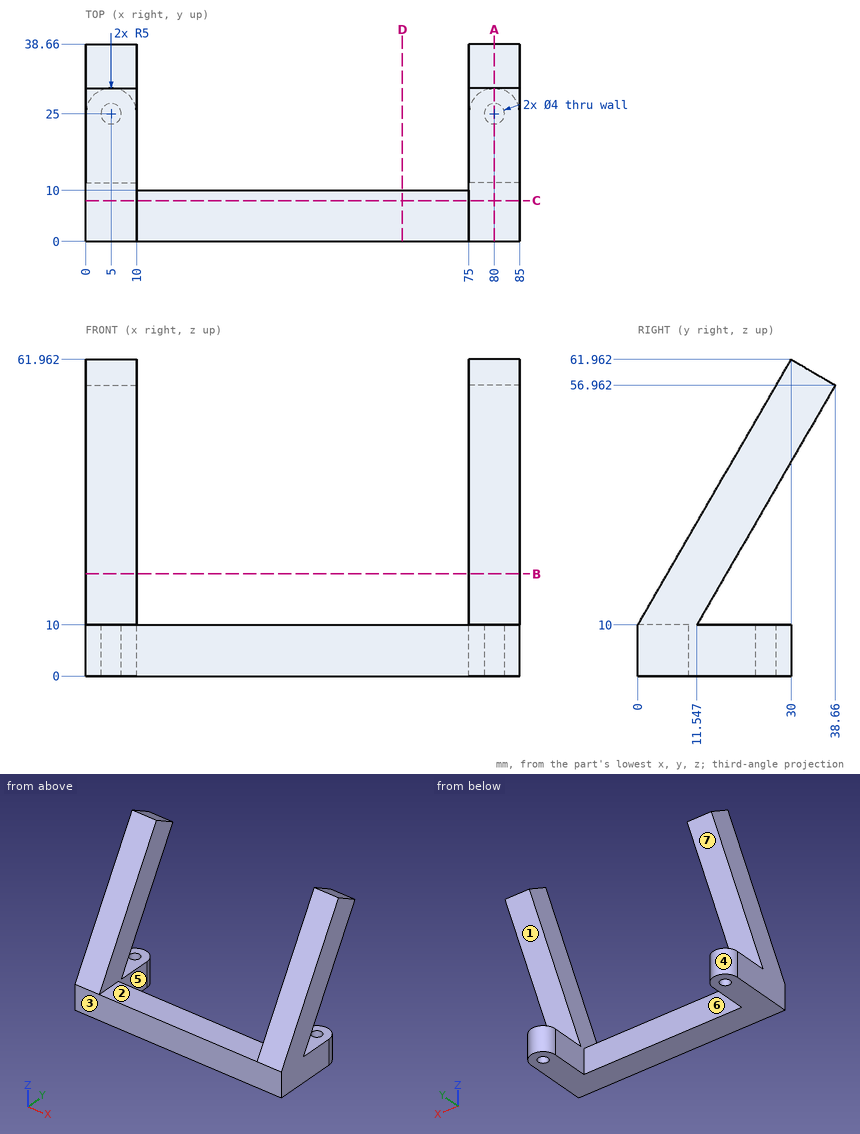
Study the drawing (mm; zero at the part's minimum x, y, z) and answer. A direction names the side the tool comes from. Coordinates: 2 decimals unless noted, no trailing zeros. Loops run counter-clockwise (first coordinate to the right, second up) from the corner with the lowest first, then second, coordinate; pieces in that order, holes last. Notation, with made-up numbers: (37.5, 35) -> (67.5, 35) arc R24 ccw to (67.5, 45) -> close; hole circle Ø8 at (66.5, 0.25). An arc over 180 degrees is marked (long way). Answer as CSV lines item,"result".
1) Flat-ended cylindrical pins translate along their axes: pin 1 (4.5 mm diameter, centred on x = 80, y = 25, fed in from +Z); pin 2 (11 mm diameter, centred on x = 43, z = 6.5, fed in from +Y); pin 3 (11 mm diameter, centred on x = 42.5, y = 3.5, fed in from +Z); pin 4 (8 mm diameter, centred on x = 38.5, z = 17.5, fed in from -Y). Find the tip coordinate at first contact, or state that the pin passes through.
A:
pin 1,"stops at z = 57.2"
pin 2,"stops at y = 10"
pin 3,"stops at z = 10"
pin 4,"passes through"
2) The part is cut by section C-C (y = 8). Give the vertices of the cut face in (x, z).
A:
outline,"(0, 0) -> (85, 0) -> (85, 23.86) -> (75, 23.86) -> (75, 10) -> (10, 10) -> (10, 23.86) -> (0, 23.86) -> close"
3) The part is cut by section D-D (x = 62). Give the vertices of the cut face in (y, z).
A:
outline,"(0, 0) -> (10, 0) -> (10, 10) -> (0, 10) -> close"
4) For a pull along Z with two mould halves and no side action, classify the marked faces 1, 2 and 3 as released by +Z, released by -Z, zero draft, split by the parting line, or undercut.
A:
face 1,"undercut"
face 2,"released by +Z"
face 3,"zero draft"
5) The part is cut by section A-A (x = 80). Give the vertices of the cut face in (y, z).
A:
outline,"(0, 0) -> (23, 0) -> (23, 10) -> (11.55, 10) -> (38.66, 56.96) -> (30, 61.96) -> (0, 10) -> close; (27, 0) -> (30, 0) -> (30, 10) -> (27, 10) -> close"
6) The part is cut by section B-B (z = 20). Give the vertices of the cut face in (x, y), and give its area (3 significant figures).
A:
outline,"(0, 5.77) -> (10, 5.77) -> (10, 17.32) -> (0, 17.32) -> close; (75, 5.77) -> (85, 5.77) -> (85, 17.32) -> (75, 17.32) -> close"
area,"231 mm²"
7) For the marked faces 4, 5, 6 and 7, determine the directions among +Z, -Z, +X, -X, +Y, -Y from which every point of the face is accessible in a straight line to the end or side of a thin tool.
A:
face 4,"-Z, +Y"
face 5,"+Z, +Y"
face 6,"+Z, -Z, +Y"
face 7,"+X, -X, +Y"
8) Straight lines are drawn through the part: probe 1 along X at (y, z) = (15.5, 9); probe 2 along Y at (x, z) = (80, 4.5); probe 3 along Z at (x, y) = (11.5, 9). For each, find the intervals that lie inside material, in ascending order.
A:
probe 1,"x = 0 to 10, 75 to 85"
probe 2,"y = 0 to 23, 27 to 30"
probe 3,"z = 0 to 10"
